from build123d import *

# Parameters (mm, degrees)
SKETCH1_R           = 10
BOSS_EXTRUDE1_DEPTH = 10


with BuildPart() as part:
    # Sketch1 → Boss-Extrude1 (new body)
    with BuildSketch(Plane.XY):
        with BuildLine():
            Line((-33.27272534, 35.670760078), (-3.27272534, 35.670760078))
            Line((-3.27272534, 35.670760078), (6.72727466, 25.670760078))
            Line((6.72727466, 25.670760078), (6.72727466, -24.329239922))
            ThreePointArc((6.72727466, -24.329239922), (9.656206848, -31.400307734), (16.72727466, -34.329239922))
            Line((16.72727466, -34.329239922), (46.72727466, -34.329239922))
            ThreePointArc((46.72727466, -34.329239922), (53.798342472, -37.258172111), (56.72727466, -44.329239922))
            Line((56.72727466, -44.329239922), (56.72727466, -64.329239922))
            Line((56.72727466, -64.329239922), (-93.27272534, -64.329239922))
            Line((-93.27272534, -64.329239922), (-93.27272534, -44.329239922))
            ThreePointArc((-93.27272534, -44.329239922), (-90.343793152, -37.258172111), (-83.27272534, -34.329239922))
            Line((-83.27272534, -34.329239922), (-53.27272534, -34.329239922))
            ThreePointArc((-53.27272534, -34.329239922), (-46.201657528, -31.400307734), (-43.27272534, -24.329239922))
            Line((-43.27272534, -24.329239922), (-43.27272534, 25.670760078))
            Line((-43.27272534, 25.670760078), (-33.27272534, 35.670760078))
        make_face()
        with Locations((-74.996311147, -50.546321168)):
            Circle(SKETCH1_R, mode=Mode.SUBTRACT)
        with Locations((40.056509267, -50.546321168)):
            Circle(SKETCH1_R, mode=Mode.SUBTRACT)
    extrude(amount=BOSS_EXTRUDE1_DEPTH)


solid = part.part
The model under review builds one solid part; all positions refer to its coordinate system, in mm. A direction names the side the tool comes from. Round coordinates to 2 decimals unless told otherwise and drop trailing zeros. Loops run counter-clockwise (first coordinate to the right, second up) from the corner with the lowest first, then second, coordinate; pieces in that order, holes last. Notation, with made-up numbers: M 0,77.5 L 11,77.5 A21 cw 11,94.5 Z; hole C 13.25,34 d1. An arc over 180 degrees is marked long. Answer as CSV lines item,"result".
1. To check wall thickness, follow L1, parallel to Y at x = -74, z = 6.25; L2, parallel to X at y = 24.5, z = 6.5; L3, parallel to Y at x = 32, z = 3.25. State the ranges of each line that lie inside material, in increasing order. Write a range as [from, to].
Outcome:
L1,"y = [-64.33, -60.5], [-40.6, -34.33]"
L2,"x = [-43.27, 6.73]"
L3,"y = [-64.33, -56.47], [-44.62, -34.33]"
2. Draft analysis for pull direction X (two halves, no side actions). For faces 4 (the face through (-65.76, -54.38, 4.93)), 5 (the face through (-17, -25, 10)), 6 (the face through (1.7, 30.7, 4.9)), state which applies: pulls with the +X half, pulls with the -X half, needs draft (parallel to the pull), parting line crosses it, or undercut.
Outcome:
face 4,"undercut"
face 5,"needs draft"
face 6,"pulls with the +X half"
3. We need section D-D (x = 34). Give the boundary of the cut face in (y, z).
Outcome:
outline,"M -64.33,0 L -58.5,0 L -58.5,10 L -64.33,10 Z; M -42.59,0 L -34.33,0 L -34.33,10 L -42.59,10 Z"
4. We need section B-B (z = 7.25). Give the boundary of the cut face in (x, y).
Outcome:
outline,"M -93.27,-64.33 L 56.73,-64.33 L 56.73,-44.33 A10 ccw 46.73,-34.33 L 16.73,-34.33 A10 cw 6.73,-24.33 L 6.73,25.67 L -3.27,35.67 L -33.27,35.67 L -43.27,25.67 L -43.27,-24.33 A10 cw -53.27,-34.33 L -83.27,-34.33 A10 ccw -93.27,-44.33 Z; hole C -75,-50.55 d20; hole C 40.06,-50.55 d20"
5. We need section C-C (y = 1). Give the boundary of the cut face in (x, z), plus the area to 3 significant figures.
Outcome:
outline,"M -43.27,0 L 6.73,0 L 6.73,10 L -43.27,10 Z"
area,"500 mm2"
6. Insertion check: pin 1 Ø2 at (x, z) = (-70.5, 3.5) entering from +Y; pin 2 Ø1.5 at (y, z) = (-42.5, 4) entering from +X; pin 3 Ø1.5 at (y, z) = (-13.5, 3) entering from -X. Each pin has a flat end and moves straight along its axis. Give the tip position at first contact, or say it passes through.
Outcome:
pin 1,"stops at y = -34.33"
pin 2,"stops at x = 56.67"
pin 3,"stops at x = -43.27"
7. We need section A-A (x = -76.5). Give the boundary of the cut face in (y, z).
Outcome:
outline,"M -64.33,0 L -60.43,0 L -60.43,10 L -64.33,10 Z; M -40.66,0 L -34.33,0 L -34.33,10 L -40.66,10 Z"
8. For faces 1 (the face through (-68, -34.329, 5)), 2 (the face through (30.066, -50.107, 4.93)), 3 (the face through (6.727, 1, 5)), list the 3-axis set-ups (+Z, -Z, +X, -X, +Y, -Y) from which the entire face can be reached by the end or side of a thin tool; tool diameter is ignored.
Outcome:
face 1,"+Z, -Z, -X, +Y"
face 2,"+Z, -Z"
face 3,"+Z, -Z, +X, +Y"
